Check sheet for the drawn part. Datum: minimum x, y, z corner. Units: mm. A direction names the side the tool comes from. Coordinates: 2 decimals unless noted, no trailing zeros. Loops run counter-clockwise (first coordinate to the right, second up) from the corner with the lowest first, then second, coordinate; pieces in that order, holes last.
Q1. Sectioned sample at D-D (x = 20). Enter the section's corners in (y, z) (1 decimal), then the cut area to 3 significant figures.
Q2. Access from +Z, -Z, +X, -X, +Y, -Y to the whole of each face (thin tool, end or side, straight path). Record for the marked faces 4, 5 and 6.
Q3. Sectioned sample at A-A (x = 24). Enter the section's corners in (y, z) (1 decimal), then the cut area to 3 significant figures.
Q4. Material ranges on probe 1 along Y at (x, z) = (20, 1.8) (1 decimal); probe 2 along Z at (x, y) = (22.5, 7); probe 3 along X at (y, z) = (15, 13), recorded low to high.
Q5. Mould release check, pull along Z, two halves, no side actions. Record for the marked faces 1, 2 and 3: +Z half, -Z half, draft (parallel to the pull), parting line (faces both ways), or undercut.
Q6. Sectioned sample at C-C (y = 19). Enter the section's corners in (x, z), then the cut area to 3 significant figures.
Q7. Sectioned sample at B-B (z = 7.5). Enter the section's corners in (x, y) (1 decimal).
Q8. Go/stop test with flat-tipped pins: P1, Ø2.5, axis at x = 16.5, z = 14, coming from the +Y side (1 decimal); P2, Ø3.5, axis at x = 38, z = 9.5, coming from the +Y side (1 decimal); P3, Ø2, axis at x = 12.5, y = 10, coming from the +Z side. Record where each tip stops, or that it passes through.
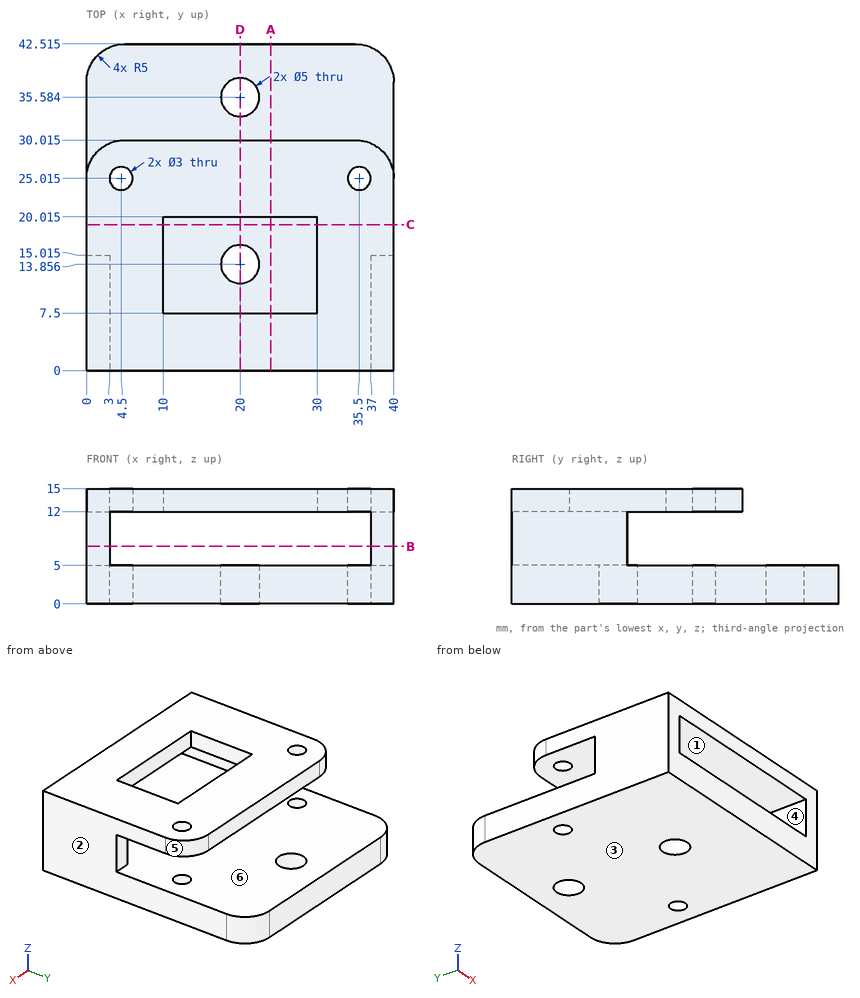
Geometry check:
1. outline: (0, 0) - (11.4, 0) - (11.4, 5) - (0, 5) - close; (0, 12) - (7.5, 12) - (7.5, 15) - (0, 15) - close; (16.4, 0) - (33.1, 0) - (33.1, 5) - (16.4, 5) - close; (20, 12) - (30, 12) - (30, 15) - (20, 15) - close; (38.1, 0) - (42.5, 0) - (42.5, 5) - (38.1, 5) - close
1. area: 215 mm2
2. face 4: +Y, -Y
2. face 5: +Z, +X, +Y
2. face 6: +Y
3. outline: (0, 0) - (42.5, 0) - (42.5, 5) - (0, 5) - close; (0, 12) - (7.5, 12) - (7.5, 15) - (0, 15) - close; (20, 12) - (30, 12) - (30, 15) - (20, 15) - close
3. area: 265 mm2
4. probe 1: y = 0 to 11.4, 16.4 to 33.1, 38.1 to 42.5
4. probe 2: z = 0 to 5, 12 to 15
4. probe 3: x = 0 to 10, 30 to 40
5. face 1: undercut
5. face 2: draft
5. face 3: -Z half
6. outline: (0, 0) - (40, 0) - (40, 5) - (0, 5) - close; (0, 12) - (10, 12) - (10, 15) - (0, 15) - close; (30, 12) - (40, 12) - (40, 15) - (30, 15) - close
6. area: 260 mm2
7. outline: (0, 0) - (3, 0) - (3, 15) - (0, 15) - close; (37, 0) - (40, 0) - (40, 15) - (37, 15) - close
8. P1: stops at y = 30
8. P2: stops at y = 15
8. P3: stops at z = 5
